Here's how the part is built. I have some questions about the finished solid (model axes, mm). A direction names the side the tool comes from. Round coordinates to 2 decimals unless told otherwise and drop trailing zeros. Write each loop counter-clockwise with the first axis right and the second up, starting at its lowest first coordinate (ties: lowest second). Pieces come first, ordered by that corner, then holes. Notation, with made-up numbers: (58, 23.5) -> (116, 23.5) arc R26 cw to (116, 39.5) -> close; hole circle Ø4 at (-9.75, -36.5). An arc over 180 degrees is marked (long way). Put each result on its own line as item: value. Start each with the question number.
1. We'd pull the mould along X, two halves only. Please class faces 5 (the face through (-64, 79.2, 99)), 6 (the face through (-27.74, -18, 99)), 7 (the face through (-54.74, -14, 99)), 8 (the face through (-66, 91.6, 99)): +X half, -X half, draft (parallel to the pull), parting line (faces both ways), or undercut.
2. I need wall thicknesses on probe 1 along X at (y, z) = (93.1, 190); probe 2 along Y at (x, z) = (-59.5, 105.5); probe 3 along Y at (x, z) = (-49, 6). Which ranges of each line are inside material? Lowest first, please. Write a range as from..to.
3. Suppose I cut it at A-A (y = 21). Please give me the cut outline in (x, z).
4. For pin 1 (1 mm diameter, centred on x = -46.5, y = 37, fed in from +Z); pin 2 (1.5 mm diameter, centred on x = -64.34, z = 6.36, fed in from +Y); pin 3 (3 mm diameter, centred on y = 50.1, z = 96, fed in from +X); pin 4 (8 mm diameter, centred on y = 75, z = 176, fed in from -X), each with a flat end and sliding along its axis, tell me the tip position at first contact or that it passes through.
5. Which directions (+Z, -Z, +X, -X, +Y, -Y) give clear straight access to the entire face, cutting with the end or side of a thin tool? Please do faces 1 (the face through (-48.052, 9.726, 124.666)), 2 (the face through (-63, 63.2, 99)), 3 (the face through (-39, 11.3, 167)), 4 (the face through (-66, -29, 99)).
```python
from build123d import *

# Parameters (mm, degrees)
RESSALTO_EXTRUS_O1_DEPTH                     = 200
CORTE_EXTRUS_O3_REACH                        = 224.463
ESBO_O4_R                                    = 1.825
CORTE_EXTRUS_O5_REACH                        = 224.463
ESBO_O6_R                                    = 6.0125
BROCA_DE_ROSQUEAR_PARA_TARRAXA_DE_M3X0_5_D   = 2.5
BROCA_DE_ROSQUEAR_PARA_TARRAXA_DE_M3_2_D     = 2.5
BROCA_DE_ROSQUEAR_PARA_TARRAXA_DE_M3_2_DEPTH = 8
BROCA_DE_ROSQUEAR_PARA_TARRAXA_DE_M3_3_D     = 2.5
BROCA_DE_ROSQUEAR_PARA_TARRAXA_DE_M3_3_DEPTH = 2
BROCA_DE_ROSQUEAR_PARA_TARRAXA_DE_M3_4_D     = 2.5
BROCA_DE_ROSQUEAR_PARA_TARRAXA_DE_M3_4_DEPTH = 2
BROCA_DE_ROSQUEAR_PARA_TARRAXA_DE_M3_5_D     = 2.5
BROCA_DE_ROSQUEAR_PARA_TARRAXA_DE_M3_5_DEPTH = 2
CORTE_EXTRUS_O6_START                        = -16.7
ESBO_O26_W                                   = 30
ESBO_O26_H                                   = 2
CORTE_EXTRUS_O6_DEPTH                        = 16.7
BROCA_DE_ROSQUEAR_PARA_TARRAXA_DE_M3_6_D     = 2.5
BROCA_DE_ROSQUEAR_PARA_TARRAXA_DE_M3_6_DEPTH = 2


with BuildPart() as part:
    # Esboço1 → Ressalto-extrusão1 (new body)
    with BuildSketch(Plane.XY):
        Polygon((-54.740307174, -0.6), (-54.740307174, 63.2), (-71.440307174, 63.2), (-71.440307174, 65.2), (-54.740307174, 65.2), (-54.740307174, 71.2), (-71.440307174, 71.2), (-71.440307174, 73.2), (-54.740307174, 73.2), (-54.740307174, 79.2), (-73.740307174, 79.2), (-73.740307174, 83), (-71.740307174, 83), (-71.740307174, 81.2), (-59.940307174, 81.2), (-59.940307174, 91.6), (-71.740307174, 91.6), (-71.740307174, 89.8), (-73.740307174, 89.8), (-73.740307174, 93.6), (-54.940307174, 93.6), (-54.940307174, 91.6), (-56.940307174, 91.6), (-56.940307174, 83.4), (-44.540307174, 83.4), (-44.540307174, 91.6), (-46.540307174, 91.6), (-46.540307174, 93.6), (-27.740307174, 93.6), (-27.740307174, 89.8), (-29.740307174, 89.8), (-29.740307174, 91.6), (-41.540307174, 91.6), (-41.540307174, 81.2), (-29.740307174, 81.2), (-29.740307174, 83), (-27.740307174, 83), (-27.740307174, 79.2), (-46.740307174, 79.2), (-46.740307174, 71.9), (-30.040307174, 71.9), (-30.040307174, 69.9), (-46.740307174, 69.9), (-46.740307174, 62.6), (-30.040307174, 62.6), (-30.040307174, 60.6), (-46.740307174, 60.6), (-46.740307174, 53.3), (-30.040307174, 53.3), (-30.040307174, 51.3), (-46.740307174, 51.3), (-46.740307174, 11.3), (-30.040307174, 11.3), (-30.040307174, 9.3), (-46.740307174, 9.3), (-46.740307174, 2), (-30.040307174, 2), (-30.040307174, 0), (-46.740307174, 0), (-46.740307174, -7.3), (-30.040307174, -7.3), (-30.040307174, -9.3), (-46.740307174, -9.3), (-46.740307174, -16.6), (-27.740307174, -16.6), (-27.740307174, -20.4), (-29.740307174, -20.4), (-29.740307174, -18.6), (-41.540307174, -18.6), (-41.540307174, -29), (-29.740307174, -29), (-29.740307174, -27.2), (-27.740307174, -27.2), (-27.740307174, -31), (-46.540307174, -31), (-46.540307174, -29), (-44.540307174, -29), (-44.540307174, -20.8), (-56.940307174, -20.8), (-56.940307174, -29), (-54.940307174, -29), (-54.940307174, -31), (-73.740307174, -31), (-73.740307174, -27.2), (-71.740307174, -27.2), (-71.740307174, -29), (-59.940307174, -29), (-59.940307174, -18.6), (-71.740307174, -18.6), (-71.740307174, -20.4), (-73.740307174, -20.4), (-73.740307174, -16.6), (-54.740307174, -16.6), (-54.740307174, -10.6), (-71.440307174, -10.6), (-71.440307174, -8.6), (-54.740307174, -8.6), (-54.740307174, -2.6), (-71.440307174, -2.6), (-71.440307174, -0.6), align=None)
    extrude(amount=RESSALTO_EXTRUS_O1_DEPTH)

    # Esboço4 → Corte-extrusão3 (cut, up to next)
    with BuildSketch(Plane.ZY.offset(54.740307174), mode=Mode.PRIVATE) as corte_extrus_o3_sk1:
        with Locations(Location((104, 50.1, 0), (0, 0, 270))):
            Circle(ESBO_O4_R)
    corte_extrus_o3_tool1 = extrude(corte_extrus_o3_sk1.sketch, amount=-CORTE_EXTRUS_O3_REACH, mode=Mode.PRIVATE) & part.part
    add(corte_extrus_o3_tool1.solids().sort_by_distance((-54.740307, 50.1, 104))[0], mode=Mode.SUBTRACT)

    # Esboço6 → Corte-extrusão5 (cut, up to next)
    with BuildSketch(Plane.ZY.offset(54.740307174), mode=Mode.PRIVATE) as corte_extrus_o5_sk1:
        with Locations(Location((130, 12.5, 0), (0, 0, 270))):
            Circle(ESBO_O6_R)
    corte_extrus_o5_tool1 = extrude(corte_extrus_o5_sk1.sketch, amount=-CORTE_EXTRUS_O5_REACH, mode=Mode.PRIVATE) & part.part
    add(corte_extrus_o5_tool1.solids().sort_by_distance((-54.740307, 12.5, 130))[0], mode=Mode.SUBTRACT)

    # Broca de rosquear para tarraxa de M3x0.5 (through all)
    with Locations(Plane.ZY.offset(54.740307174)):
        with Locations((6, 5.9), (6, 58.2)):
            Hole(BROCA_DE_ROSQUEAR_PARA_TARRAXA_DE_M3X0_5_D / 2)

    # Broca de rosquear para tarraxa de M3 2
    with Locations(Plane.ZY.offset(54.740307174)):
        with Locations((96, 50.1)):
            Hole(BROCA_DE_ROSQUEAR_PARA_TARRAXA_DE_M3_2_D / 2, depth=BROCA_DE_ROSQUEAR_PARA_TARRAXA_DE_M3_2_DEPTH)

    # Broca de rosquear para tarraxa de M3 3
    with Locations(Plane(origin=(0, 93.6, 0), x_dir=(-1, 0, 0), z_dir=(0, 1, 0))):
        with Locations((64.340307174, 190), (37.140307174, 189.76)):
            Hole(BROCA_DE_ROSQUEAR_PARA_TARRAXA_DE_M3_3_D / 2, depth=BROCA_DE_ROSQUEAR_PARA_TARRAXA_DE_M3_3_DEPTH)

    # Broca de rosquear para tarraxa de M3 4
    with Locations(Plane(origin=(0, 93.6, 0), x_dir=(-1, 0, 0), z_dir=(0, 1, 0))):
        with Locations((64.340307174, 18.36), (64.340307174, 6.36)):
            Hole(BROCA_DE_ROSQUEAR_PARA_TARRAXA_DE_M3_4_D / 2, depth=BROCA_DE_ROSQUEAR_PARA_TARRAXA_DE_M3_4_DEPTH)

    # Broca de rosquear para tarraxa de M3 5
    with Locations(Plane.XZ.offset(31)):
        with Locations((-64.340307174, 18.36), (-64.340307174, 6.36)):
            Hole(BROCA_DE_ROSQUEAR_PARA_TARRAXA_DE_M3_5_D / 2, depth=BROCA_DE_ROSQUEAR_PARA_TARRAXA_DE_M3_5_DEPTH)

    # Esboço26 → Corte-extrusão6 (cut)
    with BuildSketch(Plane(origin=(-30.040307174, 0, 0), x_dir=(0, 0, -1), z_dir=(1, 0, 0)).offset(CORTE_EXTRUS_O6_START)):
        with Locations((-105, 52.3)):
            Rectangle(ESBO_O26_W, ESBO_O26_H)
    extrude(amount=CORTE_EXTRUS_O6_DEPTH, mode=Mode.SUBTRACT)

    # Broca de rosquear para tarraxa de M3 6
    with Locations(Plane.XZ.offset(31)):
        with Locations((-64.340307174, 189.76), (-37.140307174, 189.76)):
            Hole(BROCA_DE_ROSQUEAR_PARA_TARRAXA_DE_M3_6_D / 2, depth=BROCA_DE_ROSQUEAR_PARA_TARRAXA_DE_M3_6_DEPTH)


solid = part.part
```
Verdict:
1. face 5: draft
1. face 6: +X half
1. face 7: -X half
1. face 8: undercut
2. probe 1: x = -73.74..-65.59, -63.09..-54.94, -46.54..-38.37, -35.91..-27.74
2. probe 2: y = -31..-16.6, -10.6..-8.6, -2.6..-0.6, 63.2..65.2, 71.2..73.2, 79.2..93.6
2. probe 3: y = -20.8..4.65, 7.15..56.95, 59.45..83.4
3. outline: (-54.74, 0) -> (-46.74, 0) -> (-46.74, 200) -> (-54.74, 200) -> close
4. pin 1: stops at z = 200
4. pin 2: stops at y = 81.2
4. pin 3: stops at x = -46.74
4. pin 4: stops at x = -71.44
5. face 1: +X, -X
5. face 2: +Z, -Z, -X
5. face 3: +Z, -Z, +X
5. face 4: +Z, -Z
